```python
from build123d import *

# Parameters (mm, degrees)
CROQUIS1_R              = 1.5
SALIENTE_EXTRUIR3_DEPTH = 2
CROQUIS7_W              = 20
CROQUIS7_H              = 20.25
SALIENTE_EXTRUIR4_DEPTH = 2
CROQUIS15_R             = 2
CROQUIS15_R_2           = 4
CORTAR_EXTRUIR1_DEPTH   = 10


with BuildPart() as part:
    # Croquis1 → Saliente-Extruir3 (new body)
    with BuildSketch(Plane.XY.offset(325.976420163)):
        with BuildLine():
            Line((-20.593054102, 17.650860191), (-20.593054102, -2.349139809))
            ThreePointArc((-20.593054102, -2.349139809), (-17.593054102, -5.349139809), (-14.593054102, -2.349139809))
            ThreePointArc((-14.593054102, -2.349139809), (-10.593054102, 1.650860191), (-6.593054102, -2.349139809))
            ThreePointArc((-6.593054102, -2.349139809), (-3.593054102, -5.349139809), (-0.593054102, -2.349139809))
            Line((-0.593054102, -2.349139809), (-0.593054102, 17.650860191))
            ThreePointArc((-0.593054102, 17.650860191), (-1.17884054, 19.065073753), (-2.593054102, 19.650860191))
            Line((-2.593054102, 19.650860191), (-18.593054102, 19.650860191))
            ThreePointArc((-18.593054102, 19.650860191), (-20.007267664, 19.065073753), (-20.593054102, 17.650860191))
        make_face()
        with Locations((-17.593054102, -2.349139809)):
            Circle(CROQUIS1_R, mode=Mode.SUBTRACT)
        with Locations((-10.593054102, 4.650860191)):
            Circle(CROQUIS1_R, mode=Mode.SUBTRACT)
        with Locations((-3.593054102, -2.349139809)):
            Circle(CROQUIS1_R, mode=Mode.SUBTRACT)
    extrude(amount=SALIENTE_EXTRUIR3_DEPTH)


with BuildPart() as part_1:
    # Sólido-Mover/Copiar1: read off the stored shape, not the designer's step
    # Sólido-Mover/Copiar1: moved
    add(part.part.moved(Location((0, 0, -325.9764202))))

    # Croquis7 → Saliente-Extruir4 (add)
    with BuildSketch(Plane(origin=(0, 19.650860191, 0), x_dir=(-1, 0, 0), z_dir=(0, 1, 0))):
        with Locations((10.593054102, 10.125)):
            Rectangle(CROQUIS7_W, CROQUIS7_H)
    extrude(amount=-SALIENTE_EXTRUIR4_DEPTH)

    # Simetría5: part across plane


with BuildPart() as part_2:
    add(part_1.part)
    add(part_1.part.mirror(Plane(origin=(-0.593054102, 17.650860191, 20.25), x_dir=(1, 0, 0), z_dir=(0, 0, 1))))

    # Croquis15 → Cortar-Extruir1 (cut)
    with BuildSketch(Plane(origin=(0, 19.650860191, 0), x_dir=(-1, 0, 0), z_dir=(0, 1, 0))):
        with Locations(Location((10.593054102, 27.25, 0), (0, 0, 90))):
            Circle(CROQUIS15_R)
        with Locations(Location((17.593054102, 20.25, 0), (0, 0, 90))):
            Circle(CROQUIS15_R)
        with Locations(Location((10.593054102, 13.25, 0), (0, 0, 90))):
            Circle(CROQUIS15_R)
        with Locations(Location((3.593054102, 20.25, 0), (0, 0, 90))):
            Circle(CROQUIS15_R)
        with Locations(Location((10.593054102, 20.25, 0), (0, 0, 90))):
            Circle(CROQUIS15_R_2)
    extrude(amount=-CORTAR_EXTRUIR1_DEPTH, mode=Mode.SUBTRACT)


solid = part_2.part
```
The model under review builds one solid part; all positions refer to its coordinate system, in mm. A direction names the side the tool comes from. Round coordinates to 2 decimals unless told otherwise and drop trailing zeros. Order: outer loops, then holes, each group sorted by start corner. A loop starts at its lowest first (then second) coordinate and runs counter-clockwise, first axis right, second up. Notation, with made-up numbers: (30.5, 50) -> (85.5, 50) arc R24 ccw to (85.5, 72) -> close; hole circle Ø6 at (-36.5, -26). An arc over 180 degrees is marked (long way). One line per item, written item: value. Start each with the question number.
Q1. Take a section at A-A (z = 20.25). Write out the cut boundary in (x, y), and give its area (3 significant figures).
Q2. Wall thickness on line 1 (X direction, y = 18.35, z = 20.25); line 2 (Z direction, x = -17.5, y = 11.25); line 3 (Z direction, x = -12, y = 18.5): over which ranges is each line inside the solid? List them lowest first.
Q3. Clearance check with flat-ended pins moving along their axes: pin 1 Ø2.5 at (x, z) = (-10.59, 27.25) entering from +Y; pin 2 Ø6.5 at (x, z) = (-3.59, 20.25) entering from -Y. State where each tip first meets the part, or that it passes through.
Q4. Mouldability with a two-part tool opening along Y and no side actions: class faces 3 (the face through (-13.03, 18.66, 17.08)), 4 (the face through (-4.699, -1.335, 39.514)), 5 (the face through (-3.66, -5.35, 39.51)), 6 (the face through (-10.918, 3.187, 0.986)) as released by +Y, released by -Y, zero draft, split by the parting line, or undercut.
Q5. Take a section at B-B (y = 11). Write out the cut boundary in (x, z).
Q6. Take a section at D-D (x = -13.25). Write out the cut boundary in (y, z), and give its area (3 significant figures).
Q7. Machinability: for faces 1 (the face through (-20.593, 18, 20)), 2 (the face through (-10, 17.651, 16)), which of the approach directions +Z, -Z, +X, -X, +Y, -Y give a long, thin tool a straight path to every point of the face, cutting with its end or side? Answer none if there is none.
Q8. Take a section at C-C (z = 27.25). Write out the cut boundary in (x, y).
Reported:
1. outline: (-20.59, 17.65) -> (-19.59, 17.65) -> (-19.59, 19.65) -> (-20.59, 19.65) -> close; (-15.59, 17.65) -> (-14.59, 17.65) -> (-14.59, 19.65) -> (-15.59, 19.65) -> close; (-6.59, 17.65) -> (-5.59, 17.65) -> (-5.59, 19.65) -> (-6.59, 19.65) -> close; (-1.59, 17.65) -> (-0.59, 17.65) -> (-0.59, 19.65) -> (-1.59, 19.65) -> close
1. area: 8.00 mm2
2. line 1: x = -20.59 to -19.59, -15.59 to -14.59, -6.59 to -5.59, -1.59 to -0.59
2. line 2: z = 0 to 2, 38.5 to 40.5
2. line 3: z = 0 to 11.83, 14.67 to 16.51, 23.99 to 25.83, 28.67 to 40.5
3. pin 1: passes through
3. pin 2: stops at y = 17.65
4. face 3: zero draft
4. face 4: undercut
4. face 5: released by -Y
4. face 6: undercut
5. outline: (-20.59, 0) -> (-0.59, 0) -> (-0.59, 2) -> (-20.59, 2) -> close; (-20.59, 38.5) -> (-0.59, 38.5) -> (-0.59, 40.5) -> (-20.59, 40.5) -> close
6. outline: (0.64, 0) -> (19.65, 0) -> (19.65, 17.26) -> (17.65, 17.26) -> (17.65, 2) -> (0.64, 2) -> close; (0.64, 38.5) -> (17.65, 38.5) -> (17.65, 23.24) -> (19.65, 23.24) -> (19.65, 40.5) -> (0.64, 40.5) -> close
6. area: 137 mm2
7. face 1: +Z, -Z, -X, +Y, -Y
7. face 2: +X, -X, -Y
8. outline: (-20.59, 17.65) -> (-12.59, 17.65) -> (-12.59, 19.65) -> (-20.59, 19.65) -> close; (-8.59, 17.65) -> (-0.59, 17.65) -> (-0.59, 19.65) -> (-8.59, 19.65) -> close
